```python
from build123d import *

# Parameters (mm, degrees)
F0_W     = 8.255
F0_H     = 3.81
F1_DEPTH = 25.4
F2_W     = 20.32
F2_H     = 3.81
F3_DEPTH = 12.7
F4_R     = 1.881
F5_DEPTH = 36.196
F6_R     = 1.27


with BuildPart() as f1:
    # F0 (on Top) → F1 (new body)
    with BuildSketch(Plane.XY):
        with Locations((4.1275, 1.905)):
            Rectangle(F0_W, F0_H)
        Polygon((8.255, 3.81), (8.255, 0), (12.065, 0), (12.065, 16.51), (8.255, 16.51), align=None)
        Polygon((8.255, 20.32), (8.255, 16.51), (12.065, 16.51), (32.385, 16.51), (36.195, 16.51), (36.195, 20.32), align=None)
        Polygon((36.195, 16.51), (32.385, 16.51), (32.385, 0), (36.195, 0), (36.195, 3.81), align=None)
        with Locations((40.3225, 1.905)):
            Rectangle(F0_W, F0_H)
    extrude(amount=F1_DEPTH)

    # F2 (on face) → F3 (cut)
    with BuildSketch(Plane.XY.offset(25.4)):
        with Locations((22.225, 18.415)):
            Rectangle(F2_W, F2_H)
    extrude(amount=-F3_DEPTH, mode=Mode.SUBTRACT)

    # F4 (on face) → F5 (cut, through all)
    with BuildSketch(Plane.YZ.offset(36.195)):
        with Locations((15.5575, 20.6375)):
            Circle(F4_R)
    extrude(amount=-F5_DEPTH, mode=Mode.SUBTRACT)

    # F6
    f6_edges = [f1.edges().sort_by_distance(p)[0] for p in [
        (10.16, 20.32, 25.4),
        (34.29, 20.32, 25.4),
        (22.225, 20.32, 0),
        (36.195, 20.32, 12.7),
        (8.255, 20.32, 12.7),
        (36.195, 12.065, 25.4),
        (8.255, 12.065, 25.4),
        (36.195, 12.065, 0),
        (8.255, 12.065, 0),
        (4.1275, 3.81, 0),
        (0, 3.81, 12.7),
        (4.1275, 3.81, 25.4),
        (40.3225, 3.81, 25.4),
        (44.45, 3.81, 12.7),
        (40.3225, 3.81, 0),
    ]]
    fillet(f6_edges, radius=F6_R)


solid = f1.part
```
The listing builds one solid part. Answer for the finished solid, in the listing's coordinates (mm). A direction names the side the tool comes from. Give positions to 0.01 mm unless a question says otherwise; leave off trailing zeros. Order: outer loops, then holes, each group sorted by start corner. A loop starts at its lowest first (then second) coordinate and runs counter-clockwise, first axis right, second up.
1) Find section B-B on z = 13.5. Write down the section's boundary in (x, y) (3 decimals).
Reported:
outline: (0, 0) - (12.065, 0) - (12.065, 20.32) - (9.525, 20.32) arc R1.27 ccw to (8.255, 19.05) - (8.255, 3.81) - (1.27, 3.81) arc R1.27 ccw to (0, 2.54) - close; (32.385, 0) - (44.45, 0) - (44.45, 2.54) arc R1.27 ccw to (43.18, 3.81) - (36.195, 3.81) - (36.195, 19.05) arc R1.27 ccw to (34.925, 20.32) - (32.385, 20.32) - close
2) Given P1, Ø14, axis at x = 23.5, z = 5, coming from the -Y side; P2, Ø12, axis at y = 11.5, z = 11.5, coming from the -X side (3 decimals); P3, Ø3.5, axis at y = 15.56, z = 20.64, coming from the -X side; P4, Ø2, axis at x = 38.5, z = 8.5, coming from the +Y side, each flat-ended and moving along its own axis, determine where each tip first touches the part or whether it passes through.
Reported:
P1: stops at y = 16.51
P2: stops at x = 8.255
P3: passes through
P4: stops at y = 3.81
3) For faces 1 (the face through (4.829, 3.448, 25.018)), 2 (the face through (35.81, 10.91, 0.36)), 3 (the face through (39.754, 3.448, 25.018)), determine the directions among +Z, -Z, +X, -X, +Y, -Y from which every point of the face is accessible in a straight line to the end or side of a thin tool.
Reported:
face 1: +Z, -X, +Y
face 2: -Z, +X, +Y
face 3: +Z, +X, +Y
4) Consider line 1 along X through (y, z) = (18, 16.75) (3 decimals); line 2 along Z through (x, y) = (11, 15.75); line 3 along Y through (x, z) = (28, 6.25). Determine where each line is inside the solid, lowest interval first.
Reported:
line 1: x = 8.255 to 12.065, 32.385 to 36.195
line 2: z = 0 to 18.77, 22.51 to 25.4
line 3: y = 16.51 to 20.32
5) Determine the mould class of faces 4 (the face through (44.088, 3.428, 12.878)), 5 (the face through (22, 18, 12.7)), 6 (the face through (5, 3.81, 13)) for opening direction X: pulls with the +X half, pulls with the -X half, needs draft (parallel to the pull), parting line crosses it, or undercut.
Reported:
face 4: pulls with the +X half
face 5: undercut
face 6: needs draft
6) Find section A-A on y = 8. Write down the section's boundary in (x, z) (3 decimals), then the cut area to 3 significant figures.
Reported:
outline: (8.255, 1.27) arc R1.27 ccw to (9.525, 0) - (12.065, 0) - (12.065, 25.4) - (9.525, 25.4) arc R1.27 ccw to (8.255, 24.13) - close; (32.385, 0) - (34.925, 0) arc R1.27 ccw to (36.195, 1.27) - (36.195, 24.13) arc R1.27 ccw to (34.925, 25.4) - (32.385, 25.4) - close
area: 192 mm2
7) Find section D-D on y = 16. Write down the section's boundary in (x, z) (3 decimals).
Reported:
outline: (8.255, 1.27) arc R1.27 ccw to (9.525, 0) - (12.065, 0) - (12.065, 18.809) - (8.255, 18.809) - close; (8.255, 22.466) - (12.065, 22.466) - (12.065, 25.4) - (9.525, 25.4) arc R1.27 ccw to (8.255, 24.13) - close; (32.385, 0) - (34.925, 0) arc R1.27 ccw to (36.195, 1.27) - (36.195, 18.809) - (32.385, 18.809) - close; (32.385, 22.466) - (36.195, 22.466) - (36.195, 24.13) arc R1.27 ccw to (34.925, 25.4) - (32.385, 25.4) - close
8) Find section C-C on z = 21.75. Write down the section's boundary in (x, y) (3 decimals).
Reported:
outline: (0, 0) - (12.065, 0) - (12.065, 14.041) - (8.255, 14.041) - (8.255, 3.81) - (1.27, 3.81) arc R1.27 ccw to (0, 2.54) - close; (8.255, 17.074) - (12.065, 17.074) - (12.065, 20.32) - (9.525, 20.32) arc R1.27 ccw to (8.255, 19.05) - close; (32.385, 0) - (44.45, 0) - (44.45, 2.54) arc R1.27 ccw to (43.18, 3.81) - (36.195, 3.81) - (36.195, 14.041) - (32.385, 14.041) - close; (32.385, 17.074) - (36.195, 17.074) - (36.195, 19.05) arc R1.27 ccw to (34.925, 20.32) - (32.385, 20.32) - close
